```python
from build123d import *

# Parameters (mm, degrees)
BOSS_EXTRUDE1_DEPTH                 = 130.100001
BOSS_EXTRUDE1_DEPTH_BACK            = 130.100001
SHELL1_START                        = 85.7839
SHELL1_OUTLINE_W                    = 256.200002558
SHELL1_OUTLINE_H                    = 75
SHELL1_DEPTH                        = 240.188061984
BACK_CORNER_CHAMS_SIZE              = 3
LATCH_RIB_DEPTH                     = 119.100001
LATCH_RIB_CHAMFER_SIZE              = 2.4
LPATTERN1_COUNT                     = 6
LPATTERN1_PITCH                     = 35
LATCH_RIB_CHAMFER_OF_LPATTERN1_SIZE = 2.4
STACKER_LATCH_SLOT_DEPTH            = 120.100001
STACKER_LATCH_SLOT_CHAMFER_SIZE     = 2.5
SKETCH6_W                           = 311.302660761
SKETCH6_H                           = 137.717887742
CUT_EXTRUDE1_DEPTH                  = 31
SKETCH7_W                           = 311.302660761
SKETCH7_H                           = 137.717887742
CUT_EXTRUDE2_DEPTH                  = 249.457280353


with BuildPart() as part:
    # Sketch1 → Boss-Extrude1 (new, two sides: drawn at the far end of the back side and taken through both)
    with BuildSketch(Plane(origin=(0, 0, 0), x_dir=(0, 0, -1), z_dir=(1, 0, 0)).offset(-BOSS_EXTRUDE1_DEPTH_BACK)):
        Polygon((-83.7839, 0), (-279.783940449, 0), (-325.971961984, 80), (-83.7839, 80), align=None)
    extrude(amount=BOSS_EXTRUDE1_DEPTH + BOSS_EXTRUDE1_DEPTH_BACK)

    # Shell1: read off the stored shape, not the designer's step
    # Shell1 outline → Shell1 (cut)
    with BuildSketch(Plane.XY.offset(SHELL1_START)):
        with Locations((0, 39.5)):
            Rectangle(SHELL1_OUTLINE_W, SHELL1_OUTLINE_H)
    extrude(amount=SHELL1_DEPTH, mode=Mode.SUBTRACT)

    # Back Corner Chams
    back_corner_chams_edges = [part.edges().sort_by_distance(p)[0] for p in [
        (-130.100001, 40, 83.7839),
        (130.100001, 40, 83.7839),
    ]]
    chamfer(back_corner_chams_edges, length=BACK_CORNER_CHAMS_SIZE)

    # Sketch2 → Latch Rib (add, symmetric)
    with BuildSketch(Plane(origin=(0, 0, 0), x_dir=(0, 0, -1), z_dir=(1, 0, 0))):
        Polygon((-258.783940449, 0), (-260.227316122, -2.5), (-262.915246901, -2.5), (-269.783940449, 0), align=None)
    latch_rib = extrude(amount=LATCH_RIB_DEPTH, both=True)

    # Latch Rib Chamfer
    latch_rib_chamfer_edges = [part.edges().sort_by_distance(p)[0] for p in [
        (119.100001, -2.5, 261.571281511),
        (-119.100001, -2.5, 261.571281511),
    ]]
    chamfer(latch_rib_chamfer_edges, length=LATCH_RIB_CHAMFER_SIZE)

    # LPattern1: Latch Rib ×6
    with Locations(*[(0, 0, -i * LPATTERN1_PITCH) for i in range(1, LPATTERN1_COUNT)]):
        add(latch_rib)

    # Latch Rib Chamfer of LPattern1
    latch_rib_chamfer_of_lpattern1_edges = [part.edges().sort_by_distance(p)[0] for p in [
        (119.100001, -2.5, 226.571281511),
        (-119.100001, -2.5, 226.571281511),
        (119.100001, -2.5, 191.571281511),
        (-119.100001, -2.5, 191.571281511),
        (119.100001, -2.5, 156.571281511),
        (-119.100001, -2.5, 156.571281511),
        (119.100001, -2.5, 121.571281511),
        (-119.100001, -2.5, 121.571281511),
        (119.100001, -2.5, 86.571281511),
        (-119.100001, -2.5, 86.571281511),
    ]]
    chamfer(latch_rib_chamfer_of_lpattern1_edges, length=LATCH_RIB_CHAMFER_OF_LPATTERN1_SIZE)

    # Sketch3 → Stacker Latch Slot (cut, symmetric)
    with BuildSketch(Plane(origin=(0, 0, 0), x_dir=(0, 0, -1), z_dir=(1, 0, 0))):
        Polygon((-315.971961984, 80), (-304.971961984, 80), (-307.371961984, 77.6), (-309.378016178, 77.6), align=None)
    extrude(amount=STACKER_LATCH_SLOT_DEPTH, both=True, mode=Mode.SUBTRACT)

    # Stacker Latch Slot Chamfer
    # the kernel refuses this chamfer: 2.5 mm, written as the material it adds along each edge
    with BuildSketch(Plane(origin=(120.100001, 77.6, 300.942754515), x_dir=(0, 1, 0), z_dir=(0, 0, 1))) as stacker_latch_slot_chamfer_piece_1_section:
        Polygon((STACKER_LATCH_SLOT_CHAMFER_SIZE, 0), (0, STACKER_LATCH_SLOT_CHAMFER_SIZE), (0, 0), align=None)
    stacker_latch_slot_chamfer_piece_1 = extrude(amount=19.364914362, mode=Mode.PRIVATE)
    stacker_latch_slot_chamfer_piece_1 = split(stacker_latch_slot_chamfer_piece_1, bisect_by=Plane(origin=(120.100001, 80, 300.942754515), z_dir=(0, -1, 0)), keep=Keep.TOP, mode=Mode.PRIVATE)
    add(stacker_latch_slot_chamfer_piece_1)
    with BuildSketch(Plane(origin=(-120.100001, 77.6, 300.942754515), x_dir=(0, 1, 0), z_dir=(0, 0, 1))) as stacker_latch_slot_chamfer_piece_2_section:
        Polygon((STACKER_LATCH_SLOT_CHAMFER_SIZE, 0), (0, -STACKER_LATCH_SLOT_CHAMFER_SIZE), (0, 0), align=None)
    stacker_latch_slot_chamfer_piece_2 = extrude(amount=19.364914362, mode=Mode.PRIVATE)
    stacker_latch_slot_chamfer_piece_2 = split(stacker_latch_slot_chamfer_piece_2, bisect_by=Plane(origin=(-120.100001, 80, 300.942754515), z_dir=(0, -1, 0)), keep=Keep.TOP, mode=Mode.PRIVATE)
    add(stacker_latch_slot_chamfer_piece_2)

    # LPattern2: read off the stored shape, not the designer's step
    # LPattern2: loft between two sections, ruled curve by curve
    lpattern2_from = [
        Edge.make_line((120.000001279, 80, 105.971961984), (120.000001279, 80, 94.971961984)),
        Edge.make_line((-120.000001279, 80, 94.971961984), (-120.000001279, 80, 105.971961984)),
        Edge.make_line((-120.000001279, 80, 105.971961984), (120.000001279, 80, 105.971961984)),
        Edge.make_line((120.000001279, 80, 94.971961984), (-120.000001279, 80, 94.971961984)),
    ]
    lpattern2_to = [
        Edge.make_line((117.600001279, 77.6, 99.378016178), (117.600001279, 77.6, 97.371961984)),
        Edge.make_line((-117.600001279, 77.6, 97.371961984), (-117.600001279, 77.6, 99.378016178)),
        Edge.make_line((-117.600001279, 77.6, 99.378016178), (117.600001279, 77.6, 99.378016178)),
        Edge.make_line((117.600001279, 77.6, 97.371961984), (-117.600001279, 77.6, 97.371961984)),
    ]
    lpattern2 = Solid(Shell([*[Face.make_surface_from_curves(lpattern2_from[k], lpattern2_to[k]) for k in range(4)], Face(Wire(lpattern2_from)), Face(Wire(lpattern2_to))]))
    add(lpattern2, mode=Mode.SUBTRACT)

    # LPattern2 2: loft between two sections, ruled curve by curve
    lpattern2_2_from = [
        Edge.make_line((120.000001279, 80, 140.971961984), (120.000001279, 80, 129.971961984)),
        Edge.make_line((-120.000001279, 80, 129.971961984), (-120.000001279, 80, 140.971961984)),
        Edge.make_line((-120.000001279, 80, 140.971961984), (120.000001279, 80, 140.971961984)),
        Edge.make_line((120.000001279, 80, 129.971961984), (-120.000001279, 80, 129.971961984)),
    ]
    lpattern2_2_to = [
        Edge.make_line((117.600001279, 77.6, 134.378016178), (117.600001279, 77.6, 132.371961984)),
        Edge.make_line((-117.600001279, 77.6, 132.371961984), (-117.600001279, 77.6, 134.378016178)),
        Edge.make_line((-117.600001279, 77.6, 134.378016178), (117.600001279, 77.6, 134.378016178)),
        Edge.make_line((117.600001279, 77.6, 132.371961984), (-117.600001279, 77.6, 132.371961984)),
    ]
    lpattern2_2 = Solid(Shell([*[Face.make_surface_from_curves(lpattern2_2_from[k], lpattern2_2_to[k]) for k in range(4)], Face(Wire(lpattern2_2_from)), Face(Wire(lpattern2_2_to))]))
    add(lpattern2_2, mode=Mode.SUBTRACT)

    # LPattern2 3: loft between two sections, ruled curve by curve
    lpattern2_3_from = [
        Edge.make_line((120.000001279, 80, 175.971961984), (120.000001279, 80, 164.971961984)),
        Edge.make_line((-120.000001279, 80, 164.971961984), (-120.000001279, 80, 175.971961984)),
        Edge.make_line((-120.000001279, 80, 175.971961984), (120.000001279, 80, 175.971961984)),
        Edge.make_line((120.000001279, 80, 164.971961984), (-120.000001279, 80, 164.971961984)),
    ]
    lpattern2_3_to = [
        Edge.make_line((117.600001279, 77.6, 169.378016178), (117.600001279, 77.6, 167.371961984)),
        Edge.make_line((-117.600001279, 77.6, 167.371961984), (-117.600001279, 77.6, 169.378016178)),
        Edge.make_line((-117.600001279, 77.6, 169.378016178), (117.600001279, 77.6, 169.378016178)),
        Edge.make_line((117.600001279, 77.6, 167.371961984), (-117.600001279, 77.6, 167.371961984)),
    ]
    lpattern2_3 = Solid(Shell([*[Face.make_surface_from_curves(lpattern2_3_from[k], lpattern2_3_to[k]) for k in range(4)], Face(Wire(lpattern2_3_from)), Face(Wire(lpattern2_3_to))]))
    add(lpattern2_3, mode=Mode.SUBTRACT)

    # LPattern2 4: loft between two sections, ruled curve by curve
    lpattern2_4_from = [
        Edge.make_line((120.000001279, 80, 210.971961984), (120.000001279, 80, 199.971961984)),
        Edge.make_line((-120.000001279, 80, 199.971961984), (-120.000001279, 80, 210.971961984)),
        Edge.make_line((-120.000001279, 80, 210.971961984), (120.000001279, 80, 210.971961984)),
        Edge.make_line((120.000001279, 80, 199.971961984), (-120.000001279, 80, 199.971961984)),
    ]
    lpattern2_4_to = [
        Edge.make_line((117.600001279, 77.6, 204.378016178), (117.600001279, 77.6, 202.371961984)),
        Edge.make_line((-117.600001279, 77.6, 202.371961984), (-117.600001279, 77.6, 204.378016178)),
        Edge.make_line((-117.600001279, 77.6, 204.378016178), (117.600001279, 77.6, 204.378016178)),
        Edge.make_line((117.600001279, 77.6, 202.371961984), (-117.600001279, 77.6, 202.371961984)),
    ]
    lpattern2_4 = Solid(Shell([*[Face.make_surface_from_curves(lpattern2_4_from[k], lpattern2_4_to[k]) for k in range(4)], Face(Wire(lpattern2_4_from)), Face(Wire(lpattern2_4_to))]))
    add(lpattern2_4, mode=Mode.SUBTRACT)

    # LPattern2 5: loft between two sections, ruled curve by curve
    lpattern2_5_from = [
        Edge.make_line((120.000001279, 80, 245.971961984), (120.000001279, 80, 234.971961984)),
        Edge.make_line((-120.000001279, 80, 234.971961984), (-120.000001279, 80, 245.971961984)),
        Edge.make_line((-120.000001279, 80, 245.971961984), (120.000001279, 80, 245.971961984)),
        Edge.make_line((120.000001279, 80, 234.971961984), (-120.000001279, 80, 234.971961984)),
    ]
    lpattern2_5_to = [
        Edge.make_line((117.600001279, 77.6, 239.378016178), (117.600001279, 77.6, 237.371961984)),
        Edge.make_line((-117.600001279, 77.6, 237.371961984), (-117.600001279, 77.6, 239.378016178)),
        Edge.make_line((-117.600001279, 77.6, 239.378016178), (117.600001279, 77.6, 239.378016178)),
        Edge.make_line((117.600001279, 77.6, 237.371961984), (-117.600001279, 77.6, 237.371961984)),
    ]
    lpattern2_5 = Solid(Shell([*[Face.make_surface_from_curves(lpattern2_5_from[k], lpattern2_5_to[k]) for k in range(4)], Face(Wire(lpattern2_5_from)), Face(Wire(lpattern2_5_to))]))
    add(lpattern2_5, mode=Mode.SUBTRACT)

    # LPattern2 6: loft between two sections, ruled curve by curve
    lpattern2_6_from = [
        Edge.make_line((120.000001279, 80, 280.971961984), (120.000001279, 80, 269.971961984)),
        Edge.make_line((-120.000001279, 80, 269.971961984), (-120.000001279, 80, 280.971961984)),
        Edge.make_line((-120.000001279, 80, 280.971961984), (120.000001279, 80, 280.971961984)),
        Edge.make_line((120.000001279, 80, 269.971961984), (-120.000001279, 80, 269.971961984)),
    ]
    lpattern2_6_to = [
        Edge.make_line((117.600001279, 77.6, 274.378016178), (117.600001279, 77.6, 272.371961984)),
        Edge.make_line((-117.600001279, 77.6, 272.371961984), (-117.600001279, 77.6, 274.378016178)),
        Edge.make_line((-117.600001279, 77.6, 274.378016178), (117.600001279, 77.6, 274.378016178)),
        Edge.make_line((117.600001279, 77.6, 272.371961984), (-117.600001279, 77.6, 272.371961984)),
    ]
    lpattern2_6 = Solid(Shell([*[Face.make_surface_from_curves(lpattern2_6_from[k], lpattern2_6_to[k]) for k in range(4)], Face(Wire(lpattern2_6_from)), Face(Wire(lpattern2_6_to))]))
    add(lpattern2_6, mode=Mode.SUBTRACT)

    # Sketch6 → Cut-Extrude1 (cut)
    with BuildSketch(Plane(origin=(0, 0, 83.7839), x_dir=(-1, 0, 0), z_dir=(0, 0, -1))):
        with Locations((1.437413341, 38.133965711)):
            Rectangle(SKETCH6_W, SKETCH6_H)
    extrude(amount=-CUT_EXTRUDE1_DEPTH, mode=Mode.SUBTRACT)

    # Sketch7 → Cut-Extrude2 (cut, through all)
    with BuildSketch(Plane.XY.offset(130)):
        with Locations((-1.437413341, 38.133965711)):
            Rectangle(SKETCH7_W, SKETCH7_H)
    extrude(amount=CUT_EXTRUDE2_DEPTH, mode=Mode.SUBTRACT)


solid = part.part
```
Build history of the part. All positions in model axes, mm. A direction names the side the tool comes from. Round coordinates to 2 decimals unless told otherwise and drop trailing zeros. Order: outer loops, then holes, each group sorted by start corner. A loop starts at its lowest first (then second) coordinate and runs counter-clockwise, first axis right, second up. Notation, with made-up numbers: (-33, -22) -> (-23, -22) arc R22 ccw to (-23, 7) -> close; hole circle Ø1 at (32, -13.5). An arc over 180 degrees is marked (long way). Answer in a Markdown table with one row per item.
1) Band-saw the part on A-A on y = 51. Give the cut face in (x, z), and give its area (3 significant figures).
Values:
| item | result |
|---|---|
| outline | (-130.1, 114.78) -> (-128.1, 114.78) -> (-128.1, 130) -> (-130.1, 130) -> close; (128.1, 114.78) -> (130.1, 114.78) -> (130.1, 130) -> (128.1, 130) -> close |
| area | 60.9 mm2 |
2) Wall check: L1, parallel to Y at x = -53, z = 117.5; L2, parallel to X at y = 11.5, z = 120; L3, parallel to Y at x = 104.5, z = 122. Give the ranges that are in metal, low to high.
Values:
| item | result |
|---|---|
| L1 | 0 to 2, 77 to 80 |
| L2 | -130.1 to -128.1, 128.1 to 130.1 |
| L3 | -2.5 to 2, 77 to 80 |
3) Pin check, flat tip, straight feed: P1, Ø2, axis at x = 25.5, z = 125, coming from the -Y side. Stop position of the tip, or through.
Values:
| item | result |
|---|---|
| P1 | y = -2.11 |
4) Which spindle directions (+Z, -Z, +X, -X, +Y, -Y) get a long thin tool onto all of the face, cutting with end or side? Do faces 5 (the flat face through (1, 79, 114.784)), 6 (the flat face through (128.1, 39, 122)). Say none if no direction does.
Values:
| item | result |
|---|---|
| face 5 | -Z, +X, -X, +Y, -Y |
| face 6 | +Z, -Z |
5) Mould opens along Y. For faces 1 (the flat face through (-2, 77, 122)), 2 (the flat face through (-2, 80, 122)), 3 (the flat face through (-1, 79, 130)), 4 (the flat face through (-1, 0, 118)) say: released by +Y, released by -Y, zero draft, split by the parting line, or undercut.
Values:
| item | result |
|---|---|
| face 1 | undercut |
| face 2 | released by +Y |
| face 3 | zero draft |
| face 4 | released by -Y |
6) Band-saw the part on B-B on z = 125.5. Give the cut face in (x, y).
Values:
| item | result |
|---|---|
| outline | (-130.1, 0) -> (-119.1, 0) -> (-119.1, -0.1) -> (-117.64, -1.56) -> (117.64, -1.56) -> (119.1, -0.1) -> (119.1, 0) -> (130.1, 0) -> (130.1, 80) -> (-130.1, 80) -> close; hole (-128.1, 2) -> (128.1, 2) -> (128.1, 77) -> (-128.1, 77) -> close |
